Could you check a few things on this model? Use its own coordinates, in mm. Face numbers are marked on the shaded views. A direction names the side the tool comes from. Round coordinates to 2 decimals unless told otherwise and drop trailing zeros. Loops run counter-clockwise (first coordinate to the right, second up) from the corner with the lowest first, then second, coordinate; pieces in that order, holes last. Notation, with made-up numbers: (18, 50.5) -> (36, 50.5) arc R13 cw to (36, 68.5) -> close; hole circle Ø9 at (42, 10). An arc over 180 degrees is marked (long way). One line per item, written item: value.
from build123d import *

# Parameters (mm, degrees)
BASE_FLANGE1_DEPTH      = 25
BASE_FLANGE1_DEPTH_BACK = 25
SKETCH6_R               = 1.5875
SKETCH6_R_2             = 2
CUT_EXTRUDE1_DEPTH      = 88.464278423
SKETCH7_R               = 1.984375
CUT_EXTRUDE2_DEPTH      = 10
FILLET1_R               = 3


# Sheet-metal steps are written as plain solids
with BuildPart() as part:
    # Sketch1 → Base-Flange1 (new, two sides: drawn at the far end of the back side and taken through both)
    with BuildSketch(Plane.XY.offset(-BASE_FLANGE1_DEPTH_BACK)):
        with BuildLine():
            Line((0, 80), (0, 2))
            ThreePointArc((0, 2), (0.585786438, 0.585786438), (2, 0))
            Line((2, 0), (25, 0))
            Line((25, 0), (25, -0.8))
            Line((25, -0.8), (2, -0.8))
            ThreePointArc((2, -0.8), (0.020101013, 0.020101013), (-0.8, 2))
            Line((-0.8, 2), (-0.8, 80))
            Line((-0.8, 80), (0, 80))
        make_face()
    extrude(amount=BASE_FLANGE1_DEPTH + BASE_FLANGE1_DEPTH_BACK)

    # Sketch6 → Cut-Extrude1 (cut, through all)
    with BuildSketch(Plane(origin=(0, 0, 0), x_dir=(0, 0, -1), z_dir=(1, 0, 0))):
        with Locations(Location((-5.824020981, 55.990856649, 0), (0, 0, 90))):
            Circle(SKETCH6_R)
        with Locations(Location((7.675979019, 29.2, 0), (0, 0, 90))):
            Circle(SKETCH6_R_2)
    extrude(amount=-CUT_EXTRUDE1_DEPTH, mode=Mode.SUBTRACT)

    # Sketch7 → Cut-Extrude2 (cut)
    with BuildSketch(Plane(origin=(0, 0, 0), x_dir=(1, 0, 0), z_dir=(0, 1, 0))):
        with Locations(Location((13.5, 15, 0), (0, 0, 270))):
            Circle(SKETCH7_R)
        with Locations(Location((13.5, -15, 0), (0, 0, 270))):
            Circle(SKETCH7_R)
    extrude(amount=-CUT_EXTRUDE2_DEPTH, mode=Mode.SUBTRACT)

    # Fillet1
    fillet1_edges = [part.edges().sort_by_distance(p)[0] for p in [
        (-0.4, 80, 25),
        (-0.4, 80, -25),
    ]]
    fillet(fillet1_edges, radius=FILLET1_R)


solid = part.part
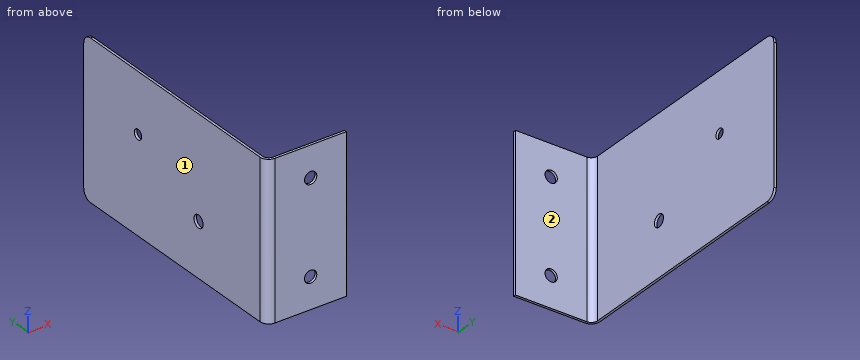
(1) If we section it at A-A, the plane z = -15: Please give me the cut outline in (x, y).
Recorded:
outline: (-0.8, 2) arc R2.8 ccw to (2, -0.8) -> (11.52, -0.8) -> (11.52, 0) -> (2, 0) arc R2 cw to (0, 2) -> (0, 80) -> (-0.8, 80) -> close; (15.48, -0.8) -> (25, -0.8) -> (25, 0) -> (15.48, 0) -> close
(2) If we section it at D-D, the plane z = -21: Please give me the cut outline in (x, y), then the cut area to 3 significant figures.
Recorded:
outline: (-0.8, 2) arc R2.8 ccw to (2, -0.8) -> (25, -0.8) -> (25, 0) -> (2, 0) arc R2 cw to (0, 2) -> (0, 80) -> (-0.8, 80) -> close
area: 83.8 mm²
(3) I'm going to push flat-ended pins straight in: pin 1 Ø1 at (y, z) = (27, 2.5) entering from +X; pin 2 Ø6.5 at (x, z) = (13.5, -15) entering from -Y; pin 3 Ø7 at (x, z) = (15, 9) entering from +Y. Where does each tip first touch, or does it pass through?
Recorded:
pin 1: x = 0
pin 2: y = -0.8
pin 3: y = 0
(4) For the marked faces 1 and 2, which set-ups out of +Z, -Z, +X, -X, +Y, -Y let a thin tool reach every point of the face, with its end or its side?
Recorded:
face 1: +Z, -Z, -X, +Y, -Y
face 2: +Z, -Z, +X, +Y
(5) If we section it at B-B, the plane y = 29.2: Please give me the cut outline in (x, z), then the cut area to 3 significant figures.
Recorded:
outline: (-0.8, -25) -> (0, -25) -> (0, -9.68) -> (-0.8, -9.68) -> close; (-0.8, -5.68) -> (0, -5.68) -> (0, 25) -> (-0.8, 25) -> close
area: 36.8 mm²
(6) If I drill on L1, parallel to Z at x = -0.6, y = 29.2; L2, parallel to Y at x = 12.25, z = -2.5, over which ranges is the centre line in solid material (lowest first)?
Recorded:
L1: -25 to -9.68, -5.68 to 25
L2: -0.8 to 0
(7) If we section it at C-C, the plane x = 13.5: Please give me the cut outline in (y, z).
Recorded:
outline: (-0.8, -25) -> (0, -25) -> (0, -16.98) -> (-0.8, -16.98) -> close; (-0.8, -13.02) -> (0, -13.02) -> (0, 13.02) -> (-0.8, 13.02) -> close; (-0.8, 16.98) -> (0, 16.98) -> (0, 25) -> (-0.8, 25) -> close
